Source: CAD feature listing. Evaluate the final solid. Frame: model axes, mm. Give positions to 0.01 mm unless a question says otherwise; leave off trailing zeros. Order: outer loops, then holes, each group sorted by start corner. A loop starts at its lowest first (then second) coordinate and runs counter-clockwise, first axis right, second up. Notation, with made-up numbers: M 86,83 L 101,83 A22 cw 101,104 Z; hole C 69,51 d3. An arc over 180 degrees is marked long. Answer in a Markdown table with one row per item. Add a question column.
(1) Material intervals for line 1 along Y through (x, z) = (-36, 1.9); line 2 along Y through (x, z) = (-21.5, 1.55); line 3 along Y through (x, z) = (-2.5, 3), sorted ascending.
(2) Section query C-C, the plane x = -14. Return loops of the section in (y, z), plus the area to 3 significant figures.
(3) Section query A-A, the plane z = 2.05. Count the separate pieces of the cut face and the enclosed holes in it, plus the area to 3 significant figures.
(4) Pin query (flat end, axial travel): P1, Ø1.5, axis at x = -6, y = 2, coming from the -Z side. Return the tip coordinate at first contact, or that it passes through.
(5) Section query B-B, the plane x = -25. Return loops of the section in (y, z), plus the area to 3 significant figures.
(6) Mould query, pull axis Y, two halves, no side actions, for faces 1 (the face through (-39.14, 5.1, 2.03)), 2 (the face through (-39.14, 0.9, 2.03)), 3 (the face through (-38.78, 3.09, 1.97)). Classes: pulls with the +Y half, pulls with the -Y half, needs draft (parallel to the pull), parting line crosses it, or undercut.
from build123d import *

# Parameters (mm, degrees)
F0_W     = 40
F0_H     = 6
F0_R     = 2
F0_R_2   = 1.875
F0_R_3   = 1.75
F0_R_4   = 1.625
F0_R_5   = 1.5
F0_R_6   = 1.375
F0_R_7   = 1.25
F1_DEPTH = 4
F2_R     = 2.99999


# Not quite as in the source:
# - a fillet or chamfer is up to 0.001 mm smaller than in the source, because OpenCascade refuses the exact size


with BuildPart() as f1:
    # F0 (on Top) → F1 (new body)
    with BuildSketch(Plane.XY):
        with Locations((-20, 3)):
            Rectangle(F0_W, F0_H)
        with Locations((-36.7836877704, 3)):
            Circle(F0_R, mode=Mode.SUBTRACT)
        with Locations((-31.2836877704, 3)):
            Circle(F0_R_2, mode=Mode.SUBTRACT)
        with Locations((-25.7836877704, 3)):
            Circle(F0_R_3, mode=Mode.SUBTRACT)
        with Locations((-20.2836877704, 3)):
            Circle(F0_R_4, mode=Mode.SUBTRACT)
        with Locations((-14.7836877704, 3)):
            Circle(F0_R_5, mode=Mode.SUBTRACT)
        with Locations((-9.2836877704, 3)):
            Circle(F0_R_6, mode=Mode.SUBTRACT)
        with Locations((-3.7836877704, 3)):
            Circle(F0_R_7, mode=Mode.SUBTRACT)
    extrude(amount=F1_DEPTH)

    # F2 (radius 3 in the source; OpenCascade refuses exactly that, so slightly less here)
    f2_edges = [f1.edges().sort_by_distance(p)[0] for p in [
        (0, 0, 2),
        (0, 6, 2),
        (-40, 0, 2),
        (-40, 6, 2),
    ]]
    fillet(f2_edges, radius=F2_R)


solid = f1.part
Values follow:
| question | item | result |
|---|---|---|
| 1 | line 1 | y = 0 to 1.16, 4.84 to 6 |
| 1 | line 2 | y = 0 to 1.92, 4.08 to 6 |
| 1 | line 3 | y = 0.04 to 5.96 |
| 2 | outline | M 0,0 L 1.72,0 L 1.72,4 L 0,4 Z; M 4.28,0 L 6,0 L 6,4 L 4.28,4 Z |
| 2 | area | 13.8 mm² |
| 3 | separate pieces | 1 |
| 3 | enclosed holes | 7 |
| 3 | area | 173 mm² |
| 4 | P1 | stops at z = 0 |
| 5 | outline | M 0,0 L 1.44,0 L 1.44,4 L 0,4 Z; M 4.56,0 L 6,0 L 6,4 L 4.56,4 Z |
| 5 | area | 11.5 mm² |
| 6 | face 1 | pulls with the +Y half |
| 6 | face 2 | pulls with the -Y half |
| 6 | face 3 | undercut |
